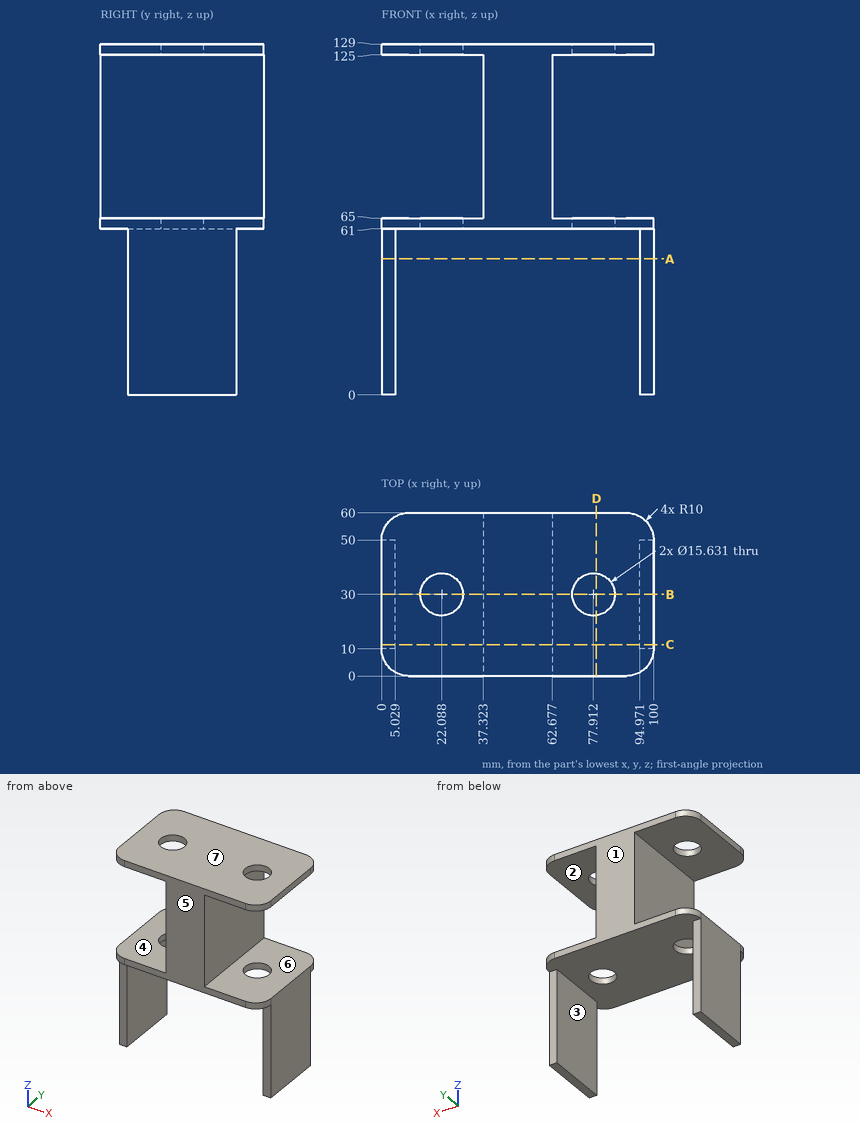
Input: dimensioned drawing with shaded views. Units: mm. Origin: part minimum x, y, z. A direction names the side the tool comes from. Give positions to 0.01 mm unless a question says otherwise; leave off trailing zeros. Write each loop counter-clockwise with the first axis right and the second up, starting at its lowest first coordinate (ties: lowest second). Pieces come first, ordered by that corner, then holes.
1. Access query for the marked faces 1, 2, 3 and 4. Directions: +Z, -Z, +X, -X, +Y, -Y. A direction counts if a zero-diameter tool reaches every point of the face in a straight line with its end or side. Return the directions, or none.
2. First-contact query: pin 1 (1.5 mm diameter, centred on x = 26, y = 34.5, fed in from +Z) (3 decimals); pin 2 (2 mm diameter, centred on x = 31, y = 22, fed in from -Z); pin 3 (5.5 mm diameter, centred on x = 2, z = 38.5, fed in from -Y); pin 4 (10 mm diameter, centred on y = 26.5, z = 92.5, fed in from -X). Flat tips, straight axial feed; report the tip coordinate or a pass-through.
3. Section query C-C (y = 11.5). Return the cut outline in (x, z).
4. Pull-direction query (Z, two-part tool) for the marked faces 5, 6 and 7; classes: +Z half, -Z half, draft (parallel to the pull), parting line (faces both ways), or undercut.
5. Material intervals for line 1 along X through (y, z) = (47, 58.5); line 2 along Z through (x, y) = (83.5, 14.5); line 3 along Z through (x, y) = (42, 51.5), sorted ascending.
6. Section query A-A (z = 50). Return the cut outline in (x, y), then the cut area to 3 significant figures.
7. Section query B-B (y = 30). Count the separate pieces of the cut face and the enclosed holes in it.
8. Section query D-D (x = 79). Return the cut outline in (y, z).
Output values:
1. face 1: +Z, -Z, +X, -X, +Y
1. face 2: +X, +Y, -Y
1. face 3: -Z, +Y, -Y
1. face 4: -X, +Y, -Y
2. pin 1: passes through
2. pin 2: stops at z = 61
2. pin 3: stops at y = 10
2. pin 4: stops at x = 37.32
3. outline: (0, 0) - (5.03, 0) - (5.03, 61) - (94.97, 61) - (94.97, 0) - (100, 0) - (100, 65) - (62.68, 65) - (62.68, 125) - (100, 125) - (100, 129) - (0, 129) - (0, 125) - (37.32, 125) - (37.32, 65) - (0, 65) - close
4. face 5: draft
4. face 6: undercut
4. face 7: +Z half
5. line 1: x = 0 to 5.03, 94.97 to 100
5. line 2: z = 61 to 65, 125 to 129
5. line 3: z = 61 to 129
6. outline: (0, 10) - (5.03, 10) - (5.03, 50) - (0, 50) - close; (94.97, 10) - (100, 10) - (100, 50) - (94.97, 50) - close
6. area: 402 mm2
7. separate pieces: 5
7. enclosed holes: 0
8. outline: (0, 61) - (22.26, 61) - (22.26, 65) - (0, 65) - close; (0, 125) - (22.26, 125) - (22.26, 129) - (0, 129) - close; (37.74, 61) - (60, 61) - (60, 65) - (37.74, 65) - close; (37.74, 125) - (60, 125) - (60, 129) - (37.74, 129) - close
